Verification items for this drawing (mm, ordinates from the low corner). A direction names the side the tool comes from. Coordinates: 2 decimals unless noted, no trailing zeros. Order: outer loops, then holes, each group sorted by start corner. A loop starts at its lowest first (then second) coordinate and runs counter-clockwise, first axis right, second up.
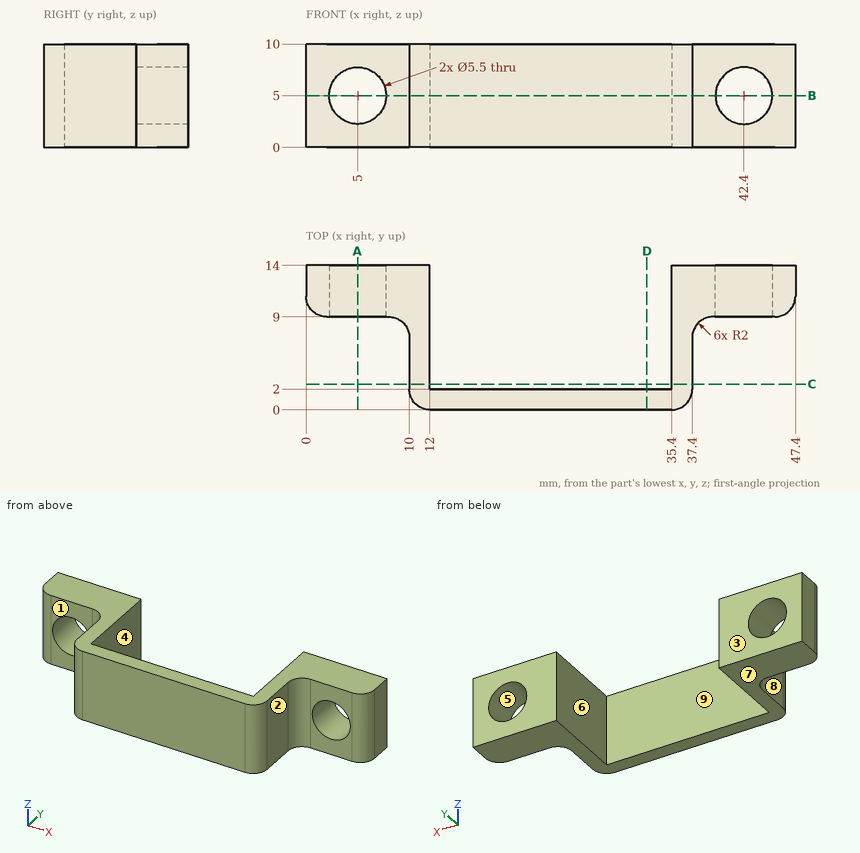
(1) Tool access check on the marked faces 1, 2, 3, 4 and 5. Record the directions out of +Z, -Z, +X, -X, +Y, -Y that give a thin tool (end or side, any length) a straight path to the whole face; none if there is none.
Filled in:
face 1: +Z, -Z, -X, -Y
face 2: +Z, -Z, +X, -Y
face 3: +Z, -Z, +X, -X, +Y
face 4: +Z, -Z, +Y
face 5: +Y, -Y
(2) Cross-section at D-D (x = 33). Enter the section's corners in (y, z).
Filled in:
outline: (0, 0) - (2, 0) - (2, 10) - (0, 10) - close
(3) Cross-section at A-A (x = 5). Enter the section's corners in (y, z), and give its area (3 significant figures).
Filled in:
outline: (9, 0) - (14, 0) - (14, 2.25) - (9, 2.25) - close; (9, 7.75) - (14, 7.75) - (14, 10) - (9, 10) - close
area: 22.5 mm2
(4) Cross-section at C-C (y = 2.5). Enter the section's corners in (x, z), and give its area (3 significant figures).
Filled in:
outline: (10, 0) - (12, 0) - (12, 10) - (10, 10) - close; (35.4, 0) - (37.4, 0) - (37.4, 10) - (35.4, 10) - close
area: 40.0 mm2
(5) Release check for a two-part mould opening along X. For the marked faces 6, 7, 8 and 9 record: +X half, -X half, draft (parallel to the pull), parting line (faces both ways), or undercut.
Filled in:
face 6: undercut
face 7: draft
face 8: -X half
face 9: undercut
(6) Thickness scan on probe 1 along X at (y, z) = (11.2, 5); probe 2 along Z at (x, y) = (42.4, 10.4); probe 3 along X at (y, z) = (5, 9). Record the ranges inside material, lowest first.
Filled in:
probe 1: x = 0 to 2.25, 7.75 to 12, 35.4 to 39.65, 45.15 to 47.4
probe 2: z = 0 to 2.25, 7.75 to 10
probe 3: x = 10 to 12, 35.4 to 37.4
(7) Go/stop test with flat-tipped pins: P1, Ø4, axis at y = 5.5, z = 6.5, coming from the +X side; P2, Ø5, axis at x = 21, z = 5, coming from the +Y side; P3, Ø5.5, axis at y = 4.5, z = 2.5, coming from the -X side; P4, Ø4, axis at x = 32.5, y = 9.5, coming from the +Z side. Record where each tip stops, or that it passes through.
Filled in:
P1: stops at x = 37.46
P2: stops at y = 2
P3: stops at x = 9.98
P4: passes through
(8) Cross-section at B-B (z = 5). Enter the section's corners in (x, y), and give its area (3 significant figures).
Filled in:
outline: (0, 11) arc R2 ccw to (2, 9) - (2.25, 9) - (2.25, 14) - (0, 14) - close; (7.75, 9) - (8, 9) arc R2 cw to (10, 7) - (10, 2) arc R2 ccw to (12, 0) - (35.4, 0) arc R2 ccw to (37.4, 2) - (37.4, 7) arc R2 cw to (39.4, 9) - (39.65, 9) - (39.65, 14) - (35.4, 14) - (35.4, 2) - (12, 2) - (12, 14) - (7.75, 14) - close; (45.15, 9) - (45.4, 9) arc R2 ccw to (47.4, 11) - (47.4, 14) - (45.15, 14) - close
area: 146 mm2
